from build123d import *

# Parameters (mm, degrees)
SKETCH2_W          = 1.583951874
SKETCH2_H          = 0.909262002
CUT_EXTRUDE1_DEPTH = 4.064


with BuildPart() as part:
    # Sketch1 → Revolve1 (revolve)
    with BuildSketch(Plane.XY, mode=Mode.PRIVATE) as revolve1_sk:
        with BuildLine():
            Line((0, 0), (12.7, 0))
            Line((12.7, 0), (12.7, 1.5875))
            Line((12.7, 1.5875), (1.5875, 1.5875))
            Line((1.5875, 1.5875), (0.3175, 2.8575))
            ThreePointArc((0.3175, 2.8575), (0.079618484, 1.437542391), (0, 0))
        make_face()
    revolve(revolve1_sk.sketch.rotate(Axis((0, 0, 0), (1, 0, 0)), 90), axis=Axis((0, 0, 0), (1, 0, 0)))

    # Sketch2 → Cut-Extrude1 (cut, symmetric)
    with BuildSketch(Plane(origin=(0, 0, 0), x_dir=(1, 0, 0), z_dir=(0, 1, 0))):
        Rectangle(SKETCH2_W, SKETCH2_H)
    extrude(amount=CUT_EXTRUDE1_DEPTH, both=True, mode=Mode.SUBTRACT)


solid = part.part
Work out the finished part from the listing and answer in its coordinate system (mm). Give positions to 0.01 mm unless a question says otherwise; leave off trailing zeros. Loops run counter-clockwise (first coordinate to the right, second up) from the corner with the lowest first, then second, coordinate; pieces in that order, holes last. Notation, with made-up numbers: (77, -23.5) -> (129, -23.5) arc R25 ccw to (129, -8.5) -> close; hole circle Ø8 at (-23.75, 10.25). An arc over 180 degrees is marked (long way). Use a Markdown table: item, result. Add a question column.
1. Flat-ended cylindrical pins translate along their axes: pin 1 Ø0.9 at (x, y) = (0.5, 1) entering from -Z; pin 2 Ø1 at (y, z) = (1.5, -2) entering from -X; pin 3 Ø2 at (y, z) = (-1.5, -1.5) entering from -X; pin 4 Ø1.5 at (y, z) = (2, -1) entering from +X. Find the tip coordinate at first contact, or state that the pin passes through.
2. Section B-B on z = 0 is taken. Determine the outline of the cut face in (x, y).
3. Find the intervals of material crossed by probe 1 along X at (y, z) = (0.2, -0.5); probe 2 along X at (y, z) = (-2, -0.5); probe 3 along Y at (x, z) = (7.75, -0.65), in increasing order.
4. Determine the mould class of faces 1 (the flat face through (0.792, 0, 0)), 2 (the conical face through (1.367, 1.765, -0.392)), 3 (the flat face through (12.7, 0, 0)) for opening direction Z: released by +Z, released by -Z, zero draft, split by the parting line, or undercut.
5. Section A-A on y = 0 is taken. Determine the outline of the cut face in (x, z) (1 decimal), and give its area (3 significant figures).
6. Section C-C on x = 7 is taken. Determine the outline of the cut face in (y, z) (1 decimal).
Results below:
| question | item | result |
|---|---|---|
| 1 | pin 1 | stops at z = -2.8 |
| 1 | pin 2 | stops at x = 0.15 |
| 1 | pin 3 | stops at x = 0.05 |
| 1 | pin 4 | stops at x = 12.7 |
| 2 | outline | (0.79, -2.38) -> (1.59, -1.59) -> (12.7, -1.59) -> (12.7, 1.59) -> (1.59, 1.59) -> (0.79, 2.38) -> close |
| 3 | probe 1 | x = 0.01 to 12.7 |
| 3 | probe 2 | x = 0.16 to 1.11 |
| 3 | probe 3 | y = -1.45 to 1.45 |
| 4 | face 1 | undercut |
| 4 | face 2 | split by the parting line |
| 4 | face 3 | zero draft |
| 5 | outline | (0, -0.5) arc R13 ccw to (0.3, -2.9) -> (1.6, -1.6) -> (12.7, -1.6) -> (12.7, 1.6) -> (1.6, 1.6) -> (0.3, 2.9) arc R13 ccw to (0, 0.5) -> (0.8, 0.5) -> (0.8, -0.5) -> close |
| 5 | area | 41.4 mm^2 |
| 6 | outline | circle Ø3.2 at (0, 0) |
